```python
from build123d import *

# Parameters (mm, degrees)
EXTRUDE_1_DEPTH     = 12
CUT_EXTRUDE_1_REACH = 111.567
SKETCH_3_R          = 3
SKETCH_5_W          = 39
SKETCH_5_H          = 3
EXTRUDE_2_DEPTH     = 18


with BuildPart() as part:
    # 草图2 → 凸台-拉伸1 (new body)
    with BuildSketch(Plane(origin=(0, 0, 0), x_dir=(0, 0, -1), z_dir=(1, 0, 0))):
        Polygon((-53, 0), (53, 0), (53, 20), (53, 22), (89, 22), (89, 25), (50, 25), (50, 20), (50, 3), (-50, 3), (-50, 14), (-53, 14), align=None)
    extrude(amount=EXTRUDE_1_DEPTH)

    # 切除-拉伸1: up to this face of the body (flat: up to its plane)
    cut_extrude_1_end = Plane(part.part.faces().sort_by_distance((6, 7, 53))[0])
    # 草图3 → 切除-拉伸1 (cut, up to the picked face)
    with BuildSketch(Plane(origin=(0, 0, -53), x_dir=(-1, 0, 0), z_dir=(0, 0, -1)), mode=Mode.PRIVATE) as cut_extrude_1_sk1:
        with Locations((-6, 14)):
            Circle(SKETCH_3_R)
    cut_extrude_1_tool1 = split(extrude(cut_extrude_1_sk1.sketch, amount=-CUT_EXTRUDE_1_REACH, mode=Mode.PRIVATE), bisect_by=cut_extrude_1_end, keep=Keep.BOTH, mode=Mode.PRIVATE)
    add(cut_extrude_1_tool1.solids().sort_by(Axis((6, 14, -53), (0, 0, 1)))[0], mode=Mode.SUBTRACT)

    # 草图5 → 凸台-拉伸2 (add)
    with BuildSketch(Plane(origin=(12, 0, 0), x_dir=(0, 0, -1), z_dir=(1, 0, 0))):
        with Locations((69.5, 23.5)):
            Rectangle(SKETCH_5_W, SKETCH_5_H)
    extrude(amount=EXTRUDE_2_DEPTH)


solid = part.part
```
For this review, take the finished solid that the model builds, in its own axes (mm). A direction names the side the tool comes from. Give positions to 0.01 mm unless a question says otherwise; leave off trailing zeros. Loops run counter-clockwise (first coordinate to the right, second up) from the corner with the lowest first, then second, coordinate; pieces in that order, holes last. Notation, with made-up numbers: M -17.5,-38 L -11.5,-38 A22 cw -11.5,-6 Z; hole C 52.5,21.25 d3. An arc over 180 degrees is marked long. One line per item, written item: value. Start each with the question number.
Q1. Add section B-B (y = 5). Give the boundary of the cut face in (x, z), and give its area (3 significant figures).
Q2. Add section D-D (y = 19.75). Give the boundary of the cut face in (x, z), and give its area (3 significant figures).
Q3. Draft analysis for pull direction Z (two halves, no side actions). For faces 1 (the face through (15, 23, -89)), 2 (the face through (6, 8, 50)), 3 (the face through (1, 14, 51)), state which applies: released by +Z, released by -Z, zero draft, split by the parting line, or undercut.
Q4. For L1, parallel to Z at x = 8.75, y = 10.5; L2, parallel to Y at x = 6, z = -50.95; L3, parallel to Y at x = 3.25, z = -16, list the stretches that pass through material, from the lowest coordinate up.
Q5. Clearance check with flat-ended pins moving along their axes: pin 1 Ø3.5 at (x, y) = (9, 10) entering from -Z; pin 2 Ø2 at (x, z) = (22.5, -60.5) entering from -Y; pin 3 Ø9.5 at (x, z) = (7, 6.5) entering from +Y. State where each tip first meets the part, or that it passes through.
Q6. Machinability: for faces 4 (the face through (12, 1, -4)), 5 (the face through (5.9, 10.8, -53)), 6 (the face through (10, 14, 51)), 7 (the face through (11, 16, -50)), which of the approach directions +Z, -Z, +X, -X, +Y, -Y give a long, thin tool a straight path to every point of the face, cutting with its end or side? Answer none if there is none.
Q7. Add section C-C (z = 22). Give the boundary of the cut face in (x, y).
Q8. Add section A-A (x = 6). Give the boundary of the cut face in (y, z), and give its area (3 significant figures).
Reply:
1. outline: M 0,-53 L 12,-53 L 12,-50 L 0,-50 Z; M 0,50 L 12,50 L 12,53 L 0,53 Z
1. area: 72.0 mm²
2. outline: M 0,-53 L 12,-53 L 12,-50 L 0,-50 Z
2. area: 36.0 mm²
3. face 1: released by -Z
3. face 2: undercut
3. face 3: zero draft
4. L1: -53 to -50, 50 to 53
4. L2: 0 to 11, 17 to 25
4. L3: 0 to 3
5. pin 1: z = -53
5. pin 2: y = 22
5. pin 3: y = 3
6. face 4: +Z, -Z, +X, -Y
6. face 5: -Z, +X, -X, -Y
6. face 6: +Z, +X, -X, +Y
6. face 7: +X, -X, +Y
7. outline: M 0,0 L 12,0 L 12,3 L 0,3 Z
8. outline: M 0,-53 L 11,-53 L 11,-50 L 3,-50 L 3,50 L 11,50 L 11,53 L 0,53 Z; M 17,-53 L 22,-53 L 22,-89 L 25,-89 L 25,-50 L 17,-50 Z
8. area: 498 mm²
